The listing builds one solid part. Answer for the finished solid, in the listing's coordinates (mm). A direction names the side the tool comes from. Give positions to 0.01 mm unless a question says otherwise; leave off trailing zeros. Write each loop counter-clockwise with the first axis right and the second up, starting at its lowest first coordinate (ties: lowest second). Pieces come first, ordered by that corner, then holes. Notation, with made-up numbers: M 55.25,21.25 L 59.25,21.25 A26 ccw 59.25,35.25 Z; hole C -32,-20 d3. An arc over 180 degrees is marked long. Answer as a JSON object with one key per item and string values.
```python
from build123d import *

# Parameters (mm, degrees)
SKETCH1_W           = 139.5
SKETCH1_H           = 152.4
BOSS_EXTRUDE1_DEPTH = 6.35
SKETCH2_W           = 139.5
SKETCH2_H           = 152.4
CUT_EXTRUDE1_DEPTH  = 3.375
SKETCH3_R           = 3.175
BOSS_EXTRUDE2_DEPTH = 12.7
SKETCH4_R           = 3.175000001
SKETCH4_R_2         = 3.175
BOSS_EXTRUDE3_DEPTH = 12.7


with BuildPart() as part:
    # Sketch1 → Boss-Extrude1 (new body)
    with BuildSketch(Plane(origin=(0, 0, 0), x_dir=(1, 0, 0), z_dir=(0, 1, 0))):
        with Locations((69.75, 76.2)):
            Rectangle(SKETCH1_W, SKETCH1_H)
    extrude(amount=BOSS_EXTRUDE1_DEPTH)

    # Sketch2 → Cut-Extrude1 (cut)
    with BuildSketch(Plane(origin=(0, 6.35, 0), x_dir=(1, 0, 0), z_dir=(0, 1, 0))):
        with Locations((69.75, 76.2)):
            Rectangle(SKETCH2_W, SKETCH2_H)
    extrude(amount=-CUT_EXTRUDE1_DEPTH, mode=Mode.SUBTRACT)

    # Sketch3 → Boss-Extrude2 (add)
    with BuildSketch(Plane.XY):
        with BuildLine():
            Line((63.4, 9.325), (63.4, 2.975))
            Line((63.4, 2.975), (76.1, 2.975))
            Line((76.1, 2.975), (76.1, 9.325000633))
            ThreePointArc((76.1, 9.325000633), (69.749999683, 15.675000317), (63.4, 9.325))
        make_face()
        with Locations((69.75, 9.325000317)):
            Circle(SKETCH3_R, mode=Mode.SUBTRACT)
    extrude(amount=-BOSS_EXTRUDE2_DEPTH)

    # Sketch4 → Boss-Extrude3 (add)
    with BuildSketch(Plane(origin=(0, 0, -152.4), x_dir=(-1, 0, 0), z_dir=(0, 0, -1))):
        with BuildLine():
            Line((-130.61, 9.325), (-130.61, 2.975))
            Line((-130.61, 2.975), (-117.91, 2.975))
            Line((-117.91, 2.975), (-117.91, 9.325))
            ThreePointArc((-117.91, 9.325), (-124.26, 15.675), (-130.61, 9.325))
        make_face()
        with Locations((-124.26, 9.325)):
            Circle(SKETCH4_R, mode=Mode.SUBTRACT)
        with BuildLine():
            Line((-21.59, 9.325), (-21.59, 2.975))
            Line((-21.59, 2.975), (-8.89, 2.975))
            Line((-8.89, 2.975), (-8.89, 9.325))
            ThreePointArc((-8.89, 9.325), (-15.24, 15.675), (-21.59, 9.325))
        make_face()
        with Locations((-15.24, 9.325)):
            Circle(SKETCH4_R_2, mode=Mode.SUBTRACT)
    extrude(amount=-BOSS_EXTRUDE3_DEPTH)


solid = part.part
```
1. Flat-ended cylindrical pins translate along their axes: pin 1 (4 mm diameter, centred on x = 127, y = 10, fed in from +Z); pin 2 (1.9 mm diameter, centred on y = 5.5, z = -8, fed in from -X); pin 3 (5 mm diameter, centred on y = 5, z = -143, fed in from -X); pin 4 (3 mm diameter, centred on y = 5.5, z = -146.5, fed in from -X). Find the tip coordinate at first contact, or state that the pin passes through.
Verdict:
{"pin 1": "stops at z = -139.7", "pin 2": "stops at x = 63.4", "pin 3": "stops at x = 0", "pin 4": "stops at x = 8.89"}
2. The mould has two halves that part along X. Classify faces 1 (the cylindrical face through (124.12, 15.673, -146.139)), 2 (the flat face through (8.89, 6, -146)), 3 (the flat face through (70, 5, -12.7)): released by +X, released by -X, zero draft, split by the parting line, or undercut.
Verdict:
{"face 1": "undercut", "face 2": "released by -X", "face 3": "zero draft"}
3. A cutting plane is placed at B-B, the plane x = 31.5. Give the vertices of the cut face in (y, z) (3 decimals), plus the area to 3 significant figures.
Verdict:
{"outline": "M 0,-152.4 L 2.975,-152.4 L 2.975,0 L 0,0 Z", "area": "453 mm2"}
4. Consider line 1 along Y through (x, z) = (15.24, -146.25) (3 decimals); line 2 along Y through (x, z) = (30.5, -14.5) (3 decimals); line 3 along X through (y, z) = (11.25, -8). Determine where each line is inside the solid, lowest interval first.
Verdict:
{"line 1": "y = 0 to 6.15, 12.5 to 15.675", "line 2": "y = 0 to 2.975", "line 3": "x = 63.7 to 67.23, 72.27 to 75.8"}
5. For faces 4 (the flat face through (63.4, 6, -6)), 5 (the flat face through (117.91, 6, -146)), 6 (the flat face through (130.61, 6, -146)), 7 (the flat face through (124, 5, -139.7)), determine the directions among +Z, -Z, +X, -X, +Y, -Y from which every point of the face is accessible in a straight line to the end or side of a thin tool.
Verdict:
{"face 4": "+Z, -Z, -X, +Y", "face 5": "+Z, -Z, +Y", "face 6": "+Z, -Z, +X, +Y", "face 7": "+Z, +X, -X, +Y"}
6. A cutting plane is placed at A-A, the plane x = 124.26. Give the vertices of the cut face in (y, z) (3 decimals), plus the area to 3 significant figures.
Verdict:
{"outline": "M 0,-152.4 L 6.15,-152.4 L 6.15,-139.7 L 2.975,-139.7 L 2.975,0 L 0,0 Z; M 12.5,-152.4 L 15.675,-152.4 L 15.675,-139.7 L 12.5,-139.7 Z", "area": "534 mm2"}
7. A cutting plane is placed at C-C, the plane z = -79.5. Give the vertices of the cut face in (x, y) (3 decimals), plus the area to 3 significant figures.
Verdict:
{"outline": "M 0,0 L 139.5,0 L 139.5,2.975 L 0,2.975 Z", "area": "415 mm2"}
